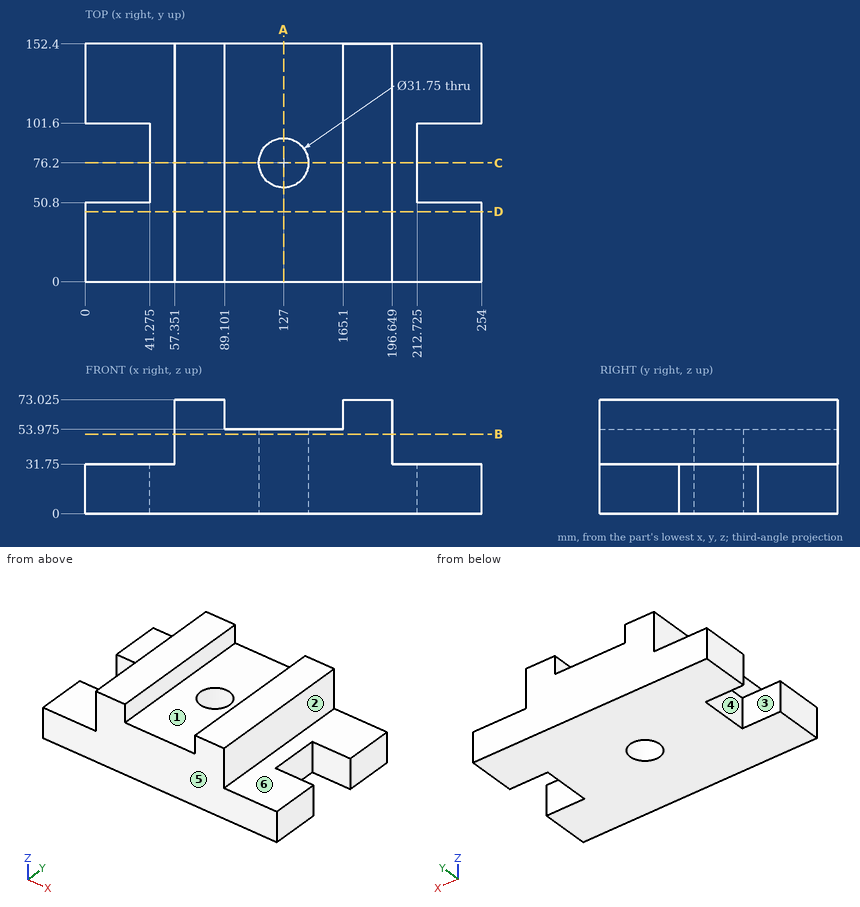
Study the drawing (mm; zero at the part's minimum x, y, z) and answer. A direction names the side the tool comes from. Give positions to 0.01 mm unless a question says otherwise; leave off trailing zeros. Write each loop counter-clockwise with the first axis right and the second up, starting at its lowest first coordinate (ties: lowest second). Pieces come first, ordered by that corner, then holes. Notation, with made-up numbers: (6.25, 6) - (24.25, 6) arc R30 cw to (24.25, 31) - close; hole circle Ø4 at (12.5, 29.5). An arc over 180 degrees is marked (long way). Use CSV: the item, a comma, the result in double quotes. Start each with the question number.
(1) Find section C-C (y = 76.2). Give the vertices of the cut face in (x, z) (3 decimals).
(2) Determine the mould class of the marked faces 4, 5 and 6 for opening direction Y: +Y half, -Y half, draft (parallel to the pull), parting line (faces both ways), or undercut.
(3) Consider line 1 along X through (y, z) = (25.5, 66.5); line 2 along X through (y, z) = (76, 16) (3 decimals); line 3 along Y through (x, z) = (127, 42.5) (3 decimals). Determine where each line is inside the solid, lowest interval first.
(4) Given P1, Ø6, axis at y = 71.5, z = 20, coming from the +X side (3 decimals); P2, Ø9.5, axis at x = 231, z = 9, coming from the -Y side; P3, Ø12.5, axis at y = 62.5, z = 59.5, coming from the +X side; P4, Ø3, axis at y = 61, z = 27, coming from the -X side (3 decimals), each flat-ended and moving along its own axis, determine where each tip first touches the part or whether it passes through.
(5) Find section B-B (z = 51). Give the vertices of the cut face in (x, y) (3 decimals), plus the area to 3 significant figures.
(6) Find section D-D (y = 45). Give the vertices of the cut face in (x, z) (3 decimals).
(7) Find section A-A (x = 127). Give the vertices of the cut face in (y, z) (3 decimals).
(8) For the marked faces 1, 2 and 3, determine the directions among +Z, -Z, +X, -X, +Y, -Y from which every point of the face is accessible in a straight line to the end or side of a thin tool.
Findings below:
1,outline,"(41.275, 0) - (111.125, 0) - (111.125, 53.975) - (89.101, 53.975) - (89.101, 73.025) - (57.351, 73.025) - (57.351, 31.75) - (41.275, 31.75) - close; (142.875, 0) - (212.725, 0) - (212.725, 31.75) - (196.649, 31.75) - (196.649, 73.025) - (165.1, 73.025) - (165.1, 53.975) - (142.875, 53.975) - close"
2,face 4,"undercut"
2,face 5,"-Y half"
2,face 6,"draft"
3,line 1,"57.35 to 89.1, 165.1 to 196.65"
3,line 2,"41.275 to 111.126, 142.874 to 212.725"
3,line 3,"0 to 60.325, 92.075 to 152.4"
4,P1,"x = 212.725"
4,P2,"y = 0"
4,P3,"x = 196.65"
4,P4,"x = 41.275"
5,outline,"(57.351, 0) - (196.649, 0) - (196.649, 152.4) - (57.351, 152.4) - close; hole circle Ø31.75 at (127, 76.2)"
5,area,"20,400 mm2"
6,outline,"(0, 0) - (254, 0) - (254, 31.75) - (196.649, 31.75) - (196.649, 73.025) - (165.1, 73.025) - (165.1, 53.975) - (89.101, 53.975) - (89.101, 73.025) - (57.351, 73.025) - (57.351, 31.75) - (0, 31.75) - close"
7,outline,"(0, 0) - (60.325, 0) - (60.325, 53.975) - (0, 53.975) - close; (92.075, 0) - (152.4, 0) - (152.4, 53.975) - (92.075, 53.975) - close"
8,face 1,"+Z, +Y, -Y"
8,face 2,"+Z, +X, +Y, -Y"
8,face 3,"+Z, -Z, -X"
